Read the model definition and answer for the solid it produces. Units are mm, in the model's axes. A direction names the side the tool comes from. Coordinates: 2 decimals unless noted, no trailing zeros. Loops run counter-clockwise (first coordinate to the right, second up) from the corner with the lowest first, then second, coordinate; pieces in that order, holes last.
from build123d import *

# Parameters (mm, degrees)
EXTRUDE_4_DEPTH     = 3
SKETCH_5_R          = 2.6
EXTRUDE_6_DEPTH     = 4.5
FILLET_1_R          = 0.5
CUT_EXTRUDE_1_DEPTH = 14.702930219


with BuildPart() as part:
    # 草图4 → 凸台-拉伸4 (new body)
    with BuildSketch(Plane.XY):
        with BuildLine():
            ThreePointArc((8.109259925, 0.007195304), (7.397764467, 0.292254868), (6.637585045, 0.390295618))
            ThreePointArc((6.637585045, 0.390295618), (6.604507127, 0.768343357), (6.549914936, 1.143888207))
            ThreePointArc((6.549914936, 1.143888207), (7.267285645, 1.413821546), (7.894339522, 1.854602872))
            ThreePointArc((7.894339522, 1.854602872), (7.809176661, 2.185613911), (7.710141023, 2.512742269))
            ThreePointArc((7.710141023, 2.512742269), (6.945380381, 2.563985838), (6.192110531, 2.422319772))
            ThreePointArc((6.192110531, 2.422319772), (6.043828385, 2.771642898), (5.875858386, 3.11193736))
            ThreePointArc((5.875858386, 3.11193736), (6.474704484, 3.590338961), (6.934859239, 4.203317219))
            ThreePointArc((6.934859239, 4.203317219), (6.751576509, 4.491810653), (6.556299797, 4.772324514))
            ThreePointArc((6.556299797, 4.772324514), (5.813134073, 4.584736009), (5.140509095, 4.217230388))
            ThreePointArc((5.140509095, 4.217230388), (4.891537611, 4.503634721), (4.626631877, 4.775368402))
            ThreePointArc((4.626631877, 4.775368402), (5.048334136, 5.415408984), (5.296546615, 6.140581589))
            ThreePointArc((5.296546615, 6.140581589), (5.033085007, 6.358317671), (4.760682268, 6.564758384))
            ThreePointArc((4.760682268, 6.564758384), (4.111857698, 6.156700276), (3.585718812, 5.599329112))
            ThreePointArc((3.585718812, 5.599329112), (3.260429054, 5.794779399), (2.924518404, 5.971353113))
            ThreePointArc((2.924518404, 5.971353113), (3.127797669, 6.710381044), (3.139771106, 7.47676305))
            ThreePointArc((3.139771106, 7.47676305), (2.821920077, 7.602428255), (2.499055988, 7.714587965))
            ThreePointArc((2.499055988, 7.714587965), (2.008084044, 7.126003823), (1.67993339, 6.433326489))
            ThreePointArc((1.67993339, 6.433326489), (1.310166985, 6.518690695), (0.936132694, 6.582820177))
            ThreePointArc((0.936132694, 6.582820177), (0.901090574, 7.348494254), (0.675652925, 8.081066849))
            ThreePointArc((0.675652925, 8.081066849), (0.334525948, 8.102360192), (-0.007195304, 8.109259925))
            ThreePointArc((-0.007195304, 8.109259925), (-0.292254868, 7.397764467), (-0.390295618, 6.637585045))
            ThreePointArc((-0.390295618, 6.637585045), (-0.768343357, 6.604507127), (-1.143888207, 6.549914936))
            ThreePointArc((-1.143888207, 6.549914936), (-1.413821546, 7.267285645), (-1.854602872, 7.894339522))
            ThreePointArc((-1.854602872, 7.894339522), (-2.185613911, 7.809176661), (-2.512742269, 7.710141023))
            ThreePointArc((-2.512742269, 7.710141023), (-2.563985838, 6.945380381), (-2.422319772, 6.192110531))
            ThreePointArc((-2.422319772, 6.192110531), (-2.771642898, 6.043828385), (-3.11193736, 5.875858386))
            ThreePointArc((-3.11193736, 5.875858386), (-3.590338961, 6.474704484), (-4.203317219, 6.934859239))
            ThreePointArc((-4.203317219, 6.934859239), (-4.491810653, 6.751576509), (-4.772324514, 6.556299797))
            ThreePointArc((-4.772324514, 6.556299797), (-4.584736009, 5.813134073), (-4.217230388, 5.140509095))
            ThreePointArc((-4.217230388, 5.140509095), (-4.503634721, 4.891537611), (-4.775368402, 4.626631877))
            ThreePointArc((-4.775368402, 4.626631877), (-5.415408984, 5.048334136), (-6.140581589, 5.296546615))
            ThreePointArc((-6.140581589, 5.296546615), (-6.358317671, 5.033085007), (-6.564758384, 4.760682268))
            ThreePointArc((-6.564758384, 4.760682268), (-6.156700276, 4.111857698), (-5.599329112, 3.585718812))
            ThreePointArc((-5.599329112, 3.585718812), (-5.794779399, 3.260429054), (-5.971353113, 2.924518404))
            ThreePointArc((-5.971353113, 2.924518404), (-6.710381044, 3.127797669), (-7.47676305, 3.139771106))
            ThreePointArc((-7.47676305, 3.139771106), (-7.602428255, 2.821920077), (-7.714587965, 2.499055988))
            ThreePointArc((-7.714587965, 2.499055988), (-7.126003823, 2.008084044), (-6.433326489, 1.67993339))
            ThreePointArc((-6.433326489, 1.67993339), (-6.518690695, 1.310166985), (-6.582820177, 0.936132694))
            ThreePointArc((-6.582820177, 0.936132694), (-7.348494254, 0.901090574), (-8.081066849, 0.675652925))
            ThreePointArc((-8.081066849, 0.675652925), (-8.102360192, 0.334525948), (-8.109259925, -0.007195304))
            ThreePointArc((-8.109259925, -0.007195304), (-7.397764467, -0.292254868), (-6.637585045, -0.390295618))
            ThreePointArc((-6.637585045, -0.390295618), (-6.604507127, -0.768343357), (-6.549914936, -1.143888207))
            ThreePointArc((-6.549914936, -1.143888207), (-7.267285646, -1.413821546), (-7.894339522, -1.854602872))
            ThreePointArc((-7.894339522, -1.854602872), (-7.809176662, -2.185613911), (-7.710141023, -2.512742269))
            ThreePointArc((-7.710141023, -2.512742269), (-6.945380381, -2.563985838), (-6.192110531, -2.422319772))
            ThreePointArc((-6.192110531, -2.422319772), (-6.043828385, -2.771642898), (-5.875858386, -3.11193736))
            ThreePointArc((-5.875858386, -3.11193736), (-6.474704484, -3.590338961), (-6.934859239, -4.203317219))
            ThreePointArc((-6.934859239, -4.203317219), (-6.751576509, -4.491810653), (-6.556299797, -4.772324514))
            ThreePointArc((-6.556299797, -4.772324514), (-5.813134073, -4.584736009), (-5.140509095, -4.217230388))
            ThreePointArc((-5.140509095, -4.217230388), (-4.891537611, -4.503634721), (-4.626631877, -4.775368402))
            ThreePointArc((-4.626631877, -4.775368402), (-5.048334136, -5.415408984), (-5.296546615, -6.140581589))
            ThreePointArc((-5.296546615, -6.140581589), (-5.033085007, -6.358317671), (-4.760682268, -6.564758384))
            ThreePointArc((-4.760682268, -6.564758384), (-4.111857698, -6.156700276), (-3.585718813, -5.599329112))
            ThreePointArc((-3.585718813, -5.599329112), (-3.260429054, -5.794779399), (-2.924518404, -5.971353114))
            ThreePointArc((-2.924518404, -5.971353114), (-3.127797669, -6.710381044), (-3.139771106, -7.47676305))
            ThreePointArc((-3.139771106, -7.47676305), (-2.821920077, -7.602428255), (-2.499055988, -7.714587965))
            ThreePointArc((-2.499055988, -7.714587965), (-2.008084044, -7.126003823), (-1.67993339, -6.433326489))
            ThreePointArc((-1.67993339, -6.433326489), (-1.310166985, -6.518690695), (-0.936132694, -6.582820177))
            ThreePointArc((-0.936132694, -6.582820177), (-0.901090574, -7.348494254), (-0.675652925, -8.081066849))
            ThreePointArc((-0.675652925, -8.081066849), (-0.334525948, -8.102360192), (0.007195304, -8.109259925))
            ThreePointArc((0.007195304, -8.109259925), (0.292254868, -7.397764467), (0.390295618, -6.637585045))
            ThreePointArc((0.390295618, -6.637585045), (0.768343357, -6.604507127), (1.143888207, -6.549914936))
            ThreePointArc((1.143888207, -6.549914936), (1.413821546, -7.267285645), (1.854602872, -7.894339522))
            ThreePointArc((1.854602872, -7.894339522), (2.185613911, -7.809176661), (2.512742269, -7.710141023))
            ThreePointArc((2.512742269, -7.710141023), (2.563985838, -6.945380381), (2.422319772, -6.192110531))
            ThreePointArc((2.422319772, -6.192110531), (2.771642898, -6.043828385), (3.11193736, -5.875858386))
            ThreePointArc((3.11193736, -5.875858386), (3.590338961, -6.474704484), (4.203317219, -6.934859239))
            ThreePointArc((4.203317219, -6.934859239), (4.491810653, -6.751576509), (4.772324514, -6.556299797))
            ThreePointArc((4.772324514, -6.556299797), (4.584736009, -5.813134073), (4.217230388, -5.140509095))
            ThreePointArc((4.217230388, -5.140509095), (4.503634721, -4.891537611), (4.775368402, -4.626631877))
            ThreePointArc((4.775368402, -4.626631877), (5.415408984, -5.048334136), (6.140581589, -5.296546615))
            ThreePointArc((6.140581589, -5.296546615), (6.358317671, -5.033085007), (6.564758384, -4.760682268))
            ThreePointArc((6.564758384, -4.760682268), (6.156700276, -4.111857698), (5.599329112, -3.585718812))
            ThreePointArc((5.599329112, -3.585718812), (5.794779399, -3.260429054), (5.971353113, -2.924518404))
            ThreePointArc((5.971353113, -2.924518404), (6.710381044, -3.127797669), (7.47676305, -3.139771106))
            ThreePointArc((7.47676305, -3.139771106), (7.602428255, -2.821920077), (7.714587965, -2.499055988))
            ThreePointArc((7.714587965, -2.499055988), (7.126003823, -2.008084044), (6.433326489, -1.67993339))
            ThreePointArc((6.433326489, -1.67993339), (6.518690695, -1.310166985), (6.582820177, -0.936132694))
            ThreePointArc((6.582820177, -0.936132694), (7.348494254, -0.901090574), (8.081066849, -0.675652925))
            ThreePointArc((8.081066849, -0.675652925), (8.102210984, -0.338120505), (8.109263117, 0))
            ThreePointArc((8.109263117, 0), (8.109262319, 0.003597652), (8.109259925, 0.007195304))
        make_face()
    extrude(amount=EXTRUDE_4_DEPTH)

    # 草图5 → 凸台-拉伸6 (add)
    with BuildSketch(Plane.XY.offset(3)):
        Circle(SKETCH_5_R)
    extrude(amount=EXTRUDE_6_DEPTH)

    # 圆角1
    fillet_1_edges = [part.edges().sort_by_distance(p)[0] for p in [
        (-2.6, 0, 7.5),
    ]]
    fillet(fillet_1_edges, radius=FILLET_1_R)

    # 草图8 → 切除-拉伸1 (cut, through all)
    with BuildSketch(Plane(origin=(0, 0, 0), x_dir=(-1, 0, 0), z_dir=(0, 0, -1))):
        with BuildLine():
            Line((0.33826518, -1.607281695), (1.534533807, 0.585648166))
            ThreePointArc((1.534533807, 0.585648166), (-1.346074271, 0.734299099), (0.33826518, -1.607281695))
        make_face()
    extrude(amount=-CUT_EXTRUDE_1_DEPTH, mode=Mode.SUBTRACT)


solid = part.part
Q1. Which of the six approach directions +Z, -Z, +X, -X, +Y, -Y give full straight-line access (tool end or side, diameter ignored) to faces 4 (the face through (-7.41, -0.29, 1.48)), 5 (the face through (2.014, 7.135, 1.479)), 6 (the face through (7.41, 0.29, 1.48)), 7 (the face through (-6.7, 3.126, 1.479))?
Findings below:
face 4: +Z, -Z, -X
face 5: +Z, -Z, +Y
face 6: +Z, -Z, +X
face 7: +Z, -Z
Q2. A cutting plane is placed at A-A (z = 5). Give the vertices of the cut face in (x, y), then the cut area to 3 significant figures.
Findings below:
outline: circle Ø5.2 at (0, 0); hole (-1.53, 0.59) - (-0.34, -1.61) arc R1.6 ccw (long way) to start
area: 14.2 mm2
Q3. Straight lines are drawn through the part: probe 1 along Y at (x, z) = (-6.25, 1.25) (3 decimals); probe 2 along Z at (x, y) = (-7, 0); probe 3 along X at (y, z) = (1, 5.5). For each, find the intervals that lie inside material, in ascending order.
Findings below:
probe 1: y = -4.719 to -3.381, -2.44 to 3.025, 4.231 to 5.167
probe 2: z = 0 to 3
probe 3: x = -2.4 to -1.28, 1.16 to 2.4
Q4. Flat-ended cylindrical pins translate along their axes: pin 1 Ø3 at (x, y) = (-0.06, -0.03) entering from -Z; pin 2 Ø8 at (x, y) = (5.5, 4) entering from +Z; pin 3 Ø3 at (x, z) = (4.5, 1.5) entering from +Y. Find the tip coordinate at first contact, or state that the pin passes through.
Findings below:
pin 1: stops at z = 0
pin 2: stops at z = 3
pin 3: stops at y = 7.53
Q5. Determine the mould class of faces 1 (the face through (-0.338, 2.578, 4.972)), 2 (the face through (-6.467, -3.583, 1.479)), 3 (the face through (4.12, 6.164, 1.479)) for opening direction Y: +Y half, -Y half, draft (parallel to the pull), parting line (faces both ways), or undercut.
Findings below:
face 1: parting line
face 2: undercut
face 3: +Y half
